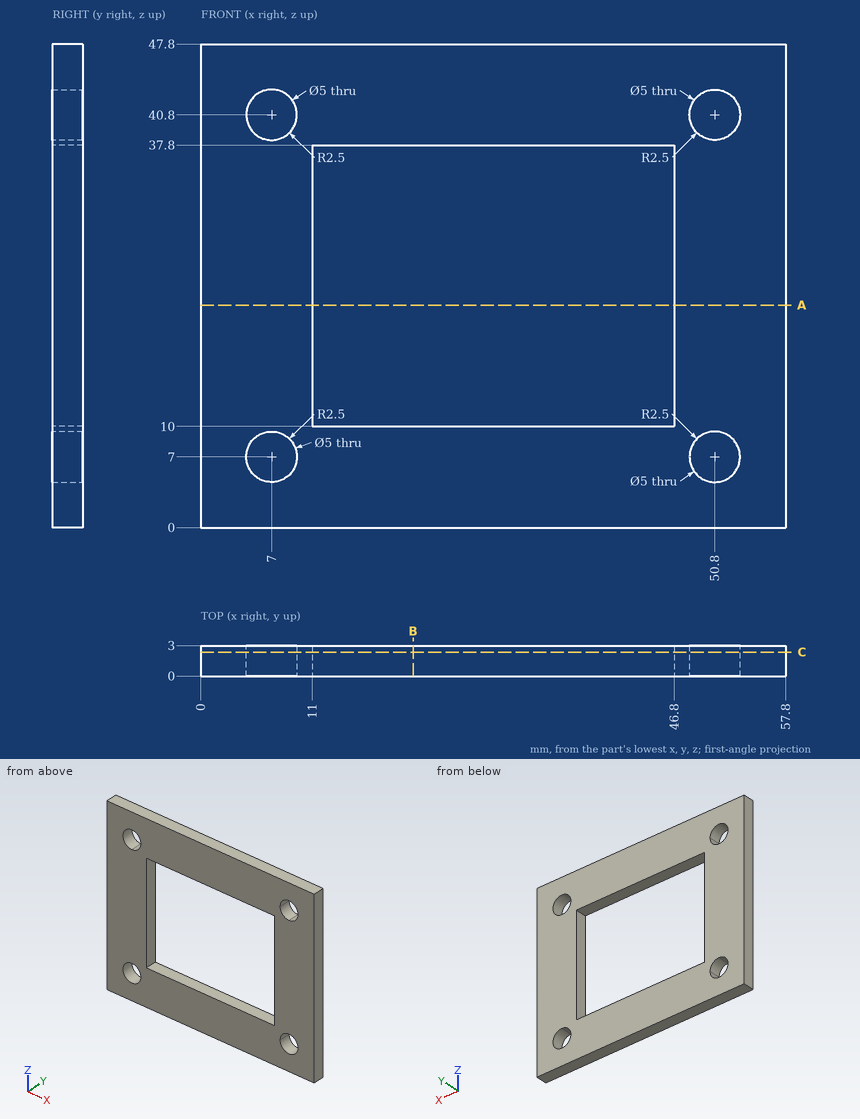
Part print with two shaded views. Sizes in mm from the minimum x, y, z corner. Coordinates: 2 decimals unless noted, no trailing zeros. Write each loop counter-clockwise with the first axis right and the second up, starting at its lowest first coordinate (ties: lowest second). Pieces come first, ordered by that corner, then holes.
(1) Drill centre lines: line 1 (Z direction, x = 50.8, y = 1.4); line 2 (X direction, y = 0.7, z = 40.8); line 3 (Z direction, x = 16.5, y = 2.6). Where is each one in solid material? Low to high.
(2) Pin check, flat tip, straight feed: pin 1 Ø4 at (x, z) = (50.8, 7) entering from -Y. Stop position of the tip, or through.
(3) Cut at A-A on z = 22. List the corners of the cut face in (x, y).
(4) Cut at C-C on y = 2.35. List the corners of the cut face in (x, z), and give its area (3 significant figures).
(5) Cut at B-B on x = 21. List the corners of the cut face in (y, z), and give its area (3 significant figures).
Working result:
1. line 1: z = 0 to 4.5, 9.5 to 38.3, 43.3 to 47.8
1. line 2: x = 0 to 4.5, 9.5 to 48.3, 53.3 to 57.8
1. line 3: z = 0 to 10, 37.8 to 47.8
2. pin 1: passes through
3. outline: (0, 0) - (11, 0) - (11, 3) - (0, 3) - close; (46.8, 0) - (57.8, 0) - (57.8, 3) - (46.8, 3) - close
4. outline: (0, 0) - (57.8, 0) - (57.8, 47.8) - (0, 47.8) - close; hole circle Ø5 at (7, 7); hole circle Ø5 at (7, 40.8); hole (11, 10) - (46.8, 10) - (46.8, 37.8) - (11, 37.8) - close; hole circle Ø5 at (50.8, 7); hole circle Ø5 at (50.8, 40.8)
4. area: 1,690 mm2
5. outline: (0, 0) - (3, 0) - (3, 10) - (0, 10) - close; (0, 37.8) - (3, 37.8) - (3, 47.8) - (0, 47.8) - close
5. area: 60.0 mm2
